Autodesk Inventor part; units mm, degrees
ref_plane "YZ Plane" through (0, 0, 0) normal (1, 0, 0) x (0, 1, 0)
ref_plane "XZ Plane" through (0, 0, 0) normal (0, 1, 0) x (-1, 0, 0)
ref_plane "XY Plane" through (0, 0, 0) normal (0, 0, 1) x (1, 0, 0)
sketch "Sketch1" plane through (0, 0, 0) normal (1, 0, 0) x (0, 1, 0)
  circle A0 centre (0, 0) radius 1.9685
  dimension "d0" = 3.937
extrude "Extrusion1" add sketch "Sketch1" along normal blind 8.636
sketch "Sketch2" plane through (8.636, 0, 0) normal (1, 0, 0) x (0, 0, -1)
  circle A0 centre (0, 0) radius 1.9685
  circle A1 centre (0, 0) radius 4.0005
  dimension "d3" = 8.001
extrude "Extrusion2" add sketch "Sketch2" along normal blind 4.191 contours A0 | A1
sketch "Sketch3" plane through (12.827, 0, 0) normal (1, 0, 0) x (0, 0, -1)
  circle A0 centre (0, 0) radius 4.0005
  circle A1 centre (0, 0) radius 3.3655
  dimension "d6" = 6.731
extrude "Extrusion3" add sketch "Sketch3" along normal blind 10.922 contours A1
sketch "Sketch4" plane through (12.827, 0, 0) normal (1, 0, 0) x (0, 0, -1)
  circle A0 centre (0, 0) radius 3.3655
  circle A1 centre (0, 0) radius 4.0005
  line L0 (-3.3655, 2.1627) -> (-3.3655, -2.1627)
  line L1 (3.3655, 2.1627) -> (3.3655, -2.1627)
extrude "Extrusion4" cut sketch "Sketch4" against normal through all contours L1 A1 | L0 A1
sketch "Sketch5" plane through (23.749, 0, 0) normal (1, 0, 0) x (0, 0, -1)
  circle A0 centre (0, 0) radius 3.3655
hole "Hole1" at (23.749, 0, 0) direction (-1, 0, 0) diameter 5.207 depth 5.08
sketch "Sketch6" plane through (18.669, 0, 0) normal (1, 0, 0) x (0, 0, -1)
  circle A0 centre (0, 0) radius 2.6035
hole "Hole2" at (18.669, 0, 0) direction (-1, 0, 0) diameter 3.937 depth 4.953
sketch "Sketch7" plane through (13.716, 0, 0) normal (1, 0, 0) x (0, 0, -1)
  circle A0 centre (0, 0) radius 1.9685
hole "Hole3" at (13.716, 0, 0) direction (-1, 0, 0) diameter 1.5748 end through all
ref_plane "Work Plane1" through (0, 0, 1.9685) normal (0, 0, 1) x (1, 0, 0)
sketch "Sketch8" plane through (0, 0, 1.9685) normal (0, 0, 1) x (1, 0, 0)
  line L0 (0, 0) -> (3.212, 0)
hole "Hole4" at (3.212, 0, 1.9685) direction (0, 0, -1) diameter 1.651 depth 1.9685
thread "Thread1"
thread "Thread2"
properties part number "Fuel Adjuster"
Can you work these out from the model? Positions are in its coordinate system, mm. A direction names the side the tool comes from. Round coordinates to 2 decimals unless told otherwise and drop trailing zeros. Write each loop counter-clockwise with the first axis right and the second up, starting at its lowest first coordinate (ties: lowest second). Pieces come first, ordered by that corner, then holes. Notation, with made-up numbers: (-37, -2.75) - (-5, -2.75) arc R20 ccw to (-5, 9.25) - close; hole circle Ø5 at (86.25, 24.25). An arc over 180 degrees is marked (long way). Write each question's results on one line, items separated by ' | '. Start each with the question number.
1) For pin 1 Ø1.2 at (y, z) = (-0.5, 1) entering from +X; pin 2 Ø1.5 at (x, y) = (4, 3) entering from +Z; pin 3 Ø1 at (y, z) = (-1.5, -1) entering from +X, each with a flat end and sliding along its axis, tell me the tip position at first contact or that it passes through.
2) Suppose I cut it at A-A (z = 0.25). List the corners of the cut face in (x, y) for me.
3) Which directions (+Z, -Z, +X, -X, +Y, -Y) give clear straight access to the entire face, cutting with the end or side of a thin tool? Please do faces 5 (the cylindrical face through (2.654, 0.608, 1.189)), 6 (the cylindrical face through (18.21, 2.05, 2.67)), 7 (the flat face through (12.827, -3.6, 0)), 8 (the cylindrical face through (4.26, -0.26, -1.95)), 9 (the flat face through (12.827, 3.5, 0.5)).
4) Suppose I cut it at B-B (x = 19.25). List the corners of the cut face in (y, z) for me, and give its area (3 significant figures).
5) We'd pull the mould along Z, two halves only. Please class faces 1 (the flat face through (18.669, -2, 1)), 2 (the flat face through (23.749, -2, -2)), 3 (the cylindrical face through (16.16, 1.92, 0.43)), 4 (the flat face through (11, 0, -3.366)): released by +Z, released by -Z, zero draft, split by the parting line, or undercut.
6) Suppose I cut it at C-C (y = 1.75). List the corners of the cut face in (x, z) for me.
7) Suppose I cut it at D-D (z = -1.75). List the corners of the cut face in (x, y) for me, and give its area (3 significant figures).
8) Please list where these lines run through material, in increasing order: line 1 (Z direction, x = 5, y = 0); line 2 (Z direction, x = 21.85, y = 0); line 3 (X direction, y = 0, z = 1.1).
Here are the results:
1) pin 1: stops at x = 13.72 | pin 2: passes through | pin 3: stops at x = 18.67
2) outline: (0, -1.95) - (8.64, -1.95) - (8.64, -3.99) - (12.83, -3.99) - (12.83, -3.36) - (23.75, -3.36) - (23.75, -2.59) - (18.67, -2.59) - (18.67, -1.95) - (13.72, -1.95) - (13.72, -0.75) - (3.56, -0.75) arc R0.83 cw to (2.86, -0.75) - (0, -0.75) - close; (0, 0.75) - (2.86, 0.75) arc R0.83 cw to (3.56, 0.75) - (13.72, 0.75) - (13.72, 1.95) - (18.67, 1.95) - (18.67, 2.59) - (23.75, 2.59) - (23.75, 3.36) - (12.83, 3.36) - (12.83, 3.99) - (8.64, 3.99) - (8.64, 1.95) - (0, 1.95) - close
3) face 5: +Z | face 6: +X | face 7: +X, -Y | face 8: -X | face 9: +X, +Y
4) outline: circle Ø6.73 at (0, 0); hole circle Ø5.21 at (0, 0) | area: 14.3 mm2
5) face 1: undercut | face 2: zero draft | face 3: undercut | face 4: released by -Z
6) outline: (0, -0.9) - (8.64, -0.9) - (8.64, -3.37) - (12.83, -3.37) - (12.83, -2.87) - (23.75, -2.87) - (23.75, -1.93) - (18.67, -1.93) - (18.67, -0.9) - (13.72, -0.9) - (13.72, 0.9) - (18.67, 0.9) - (18.67, 1.93) - (23.75, 1.93) - (23.75, 2.87) - (12.83, 2.87) - (12.83, 3.37) - (8.64, 3.37) - (8.64, 0.9) - (0, 0.9) - close
7) outline: (0, -0.9) - (8.64, -0.9) - (8.64, -3.6) - (12.83, -3.6) - (12.83, -2.87) - (23.75, -2.87) - (23.75, -1.93) - (18.67, -1.93) - (18.67, -0.9) - (13.72, -0.9) - (13.72, 0.9) - (18.67, 0.9) - (18.67, 1.93) - (23.75, 1.93) - (23.75, 2.87) - (12.83, 2.87) - (12.83, 3.6) - (8.64, 3.6) - (8.64, 0.9) - (0, 0.9) - close | area: 80.0 mm2
8) line 1: z = -1.97 to -0.79, 0.79 to 1.97 | line 2: z = -3.37 to -2.6, 2.6 to 3.37 | line 3: x = 0 to 2.39, 4.04 to 13.72
